Here's the drawing with two shaded views (mm, measured from the low corner). I have some questions. Coordinates: 2 decimals unless noted, no trailing zeros. Order: outer loops, then holes, each group sorted by start corner. A loop starts at its lowest first (then second) coordinate and runs counter-clockwise, first axis right, second up. Notation, with made-up numbers: (25.25, 43) -> (66.25, 43) arc R21 ccw to (66.25, 50) -> close; hole circle Ø1 at (81.25, 11.25). An arc over 180 degrees is marked (long way). Return JSON: item names as keys, results as strings. Group by question number.
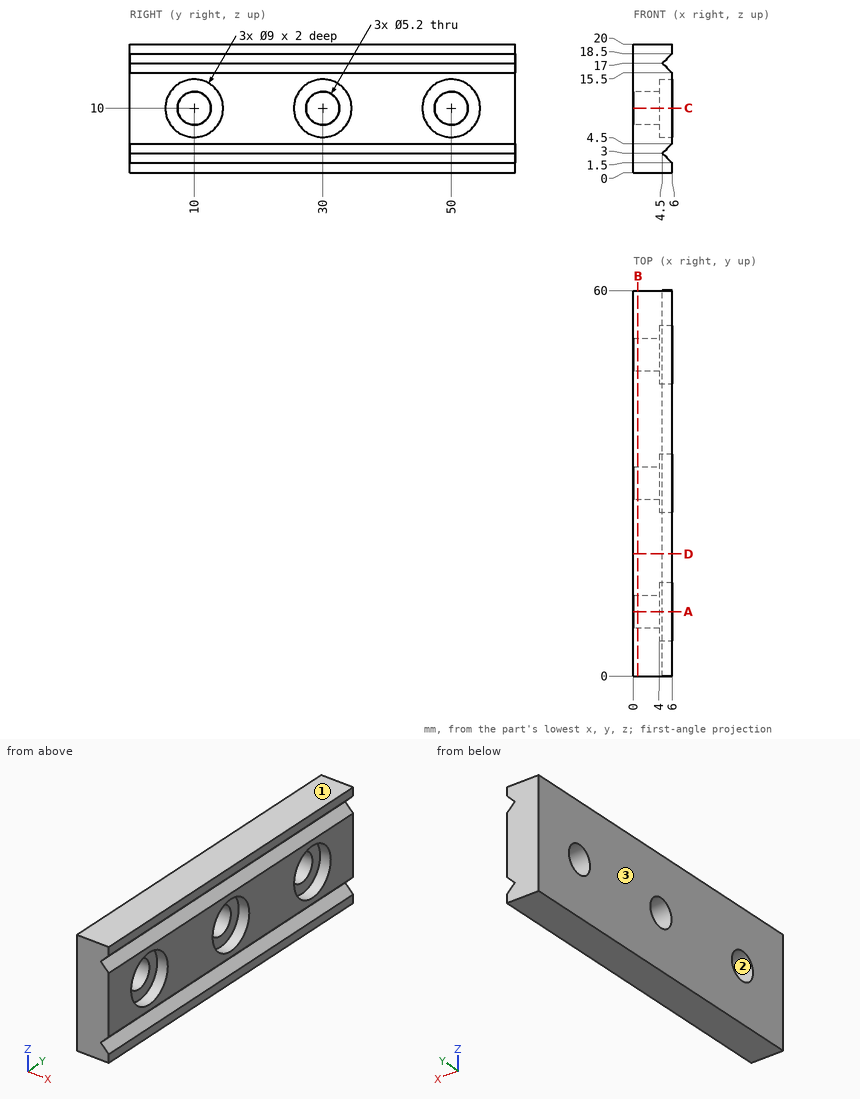
Q1. I need wall thicknesses on line 1 along Y through (x, z) = (3, 10.25); line 2 along Z through (x, y) = (4.7, 30); line 3 along Y through (x, z) = (5.1, 13.75). Which ranges of each line are inside material? Lowest first, please. Write a range as from..to.
Q2. I want a section at D-D on y = 19. Please give me the cut outline in (x, z), and give its area (4 significant figures).
Q3. I'm going to push a flat-ended pin straight in: pin 1 Ø5.5 at (y, z) = (50, 10) entering from +X. Where does the tip first touch, or does it pass through?
Q4. I want a section at C-C on z = 10. Please give me the cut outline in (x, y), and give its area (3 significant figures).
Q5. We'd pull the mould along Z, two halves only. Please class the marked faces 1, 2 and 3: pulls with the +Z half, pulls with the -Z half, needs draft (parallel to the pull), parting line crosses it, or undercut.
Q6. I want a section at B-B on x = 0.7. Please give me the cut outline in (y, z).
Q7. I want a section at A-A on y = 10. Please give me the cut outline in (x, z).
Response values:
{
 "1": {"line 1": "y = 0..7.41, 12.59..27.41, 32.59..47.41, 52.59..60", "line 2": "z = 0..2.8, 3.2..5.5, 14.5..16.8, 17.2..20", "line 3": "y = 0..7.51, 12.49..27.51, 32.49..47.51, 52.49..60"},
 "2": {"outline": "(0, 0) -> (6, 0) -> (6, 1.5) -> (4.5, 3) -> (6, 4.5) -> (6, 15.5) -> (4.5, 17) -> (6, 18.5) -> (6, 20) -> (0, 20) -> close", "area": "115.5 mm²"},
 "3": {"pin 1": "stops at x = 4"},
 "4": {"outline": "(0, 0) -> (6, 0) -> (6, 5.5) -> (4, 5.5) -> (4, 7.4) -> (0, 7.4) -> close; (0, 12.6) -> (4, 12.6) -> (4, 14.5) -> (6, 14.5) -> (6, 25.5) -> (4, 25.5) -> (4, 27.4) -> (0, 27.4) -> close; (0, 32.6) -> (4, 32.6) -> (4, 34.5) -> (6, 34.5) -> (6, 45.5) -> (4, 45.5) -> (4, 47.4) -> (0, 47.4) -> close; (0, 52.6) -> (4, 52.6) -> (4, 54.5) -> (6, 54.5) -> (6, 60) -> (0, 60) -> close", "area": "244 mm²"},
 "5": {"face 1": "pulls with the +Z half", "face 2": "undercut", "face 3": "needs draft"},
 "6": {"outline": "(0, 0) -> (60, 0) -> (60, 20) -> (0, 20) -> close; hole circle Ø5.2 at (10, 10); hole circle Ø5.2 at (30, 10); hole circle Ø5.2 at (50, 10)"},
 "7": {"outline": "(0, 0) -> (6, 0) -> (6, 1.5) -> (4.5, 3) -> (6, 4.5) -> (6, 5.5) -> (4, 5.5) -> (4, 7.4) -> (0, 7.4) -> close; (0, 12.6) -> (4, 12.6) -> (4, 14.5) -> (6, 14.5) -> (6, 15.5) -> (4.5, 17) -> (6, 18.5) -> (6, 20) -> (0, 20) -> close"}
}
